Could you check a few things on this model? Use its own coordinates, in mm. A direction names the side the tool comes from. Round coordinates to 2 decimals unless told otherwise and drop trailing zeros. Order: outer loops, then holes, each group sorted by start corner. A loop starts at its lowest first (then second) coordinate and runs counter-clockwise, first axis right, second up. Notation, with made-up numbers: M 80,79.25 L 86,79.25 A17 cw 86,110.25 Z; hole C 69.25,-35.5 d10. An arc over 180 degrees is marked long. Write each question's results on one line, items separated by ' | '. Start each with the question number.
1. We'd pull the mould along Y, two halves only. Please class faces 3 (the flat face through (-7.8, 57.8, -3.9)), 4 (the flat face through (0, 122, -2)), 5 (the flat face through (-71, 240, -2)): released by +Y, released by -Y, zero draft, split by the parting line, or undercut.
2. Suppose I cut it at A-A on z = -1. Give the number of separate pieces and of enclosed holes in the cut face, and give its area (3 significant figures).
3. Please list where these lines run through material, in increasing order: L1, parallel to X at y = 180, z = -2.1; L2, parallel to X at y = 180, z = -4.5; L3, parallel to Y at x = -54.5, z = -1.35.
4. I'm going to push a flat-ended pin straight in: pin 1 (5 mm diameter, centred on x = -69, y = 10, fed in from +Z). Where does the tip first touch, or does it pass through?
5. For faces 1 (the cylindrical face through (-71.5, 225.23, -1.98)), 2 (the cylindrical face through (-71.432, 190.906, -2.465)), which set-ups out of +Z, -Z, +X, -X, +Y, -Y let a thin tool reach every point of the face, with its end or its side?
6. Suppose I cut it at B-B on y = 230. Write out the boundary of the cut face in (x, z), and give its area (3 significant figures).
Autodesk Inventor part; units mm, degrees
ref_plane "Arbeitsebene1" through (-140, 120, 0) normal (0, 1, 0) x (1, 0, 0)
ref_plane "YZ Plane" through (0, 0, 0) normal (1, 0, 0) x (0, 1, 0)
ref_plane "XZ Plane" through (0, 0, 0) normal (0, 1, 0) x (-1, 0, 0)
sketch "Skizze3" plane through (0, 0, 0) normal (0, 0, 1) x (1, 0, 0)
  line L0 (0, 0) -> (-140, 0)
  line L1 (-140, 0) -> (-140, 120)
  line L2 (-140, 240) -> (0, 240)
  line L3 (0, 240) -> (0, 0)
  line L4 (-34.5565, 44.5) -> (-109.2584, 44.5) construction
  line L5 (-42.5521, 75.5) -> (-110.6291, 75.5) construction
  line L6 (-85.5, 104.3529) -> (-85.5, 36.2759) construction
  line L7 (-54.5, 102.2969) -> (-54.5, 32.1639) construction
  line L8 (-70, -15.9958) -> (-70, 12.0858) construction
  circle A0 centre (-70, 60) radius 11
  circle A1 centre (-85.5, 75.5) radius 1.5
  circle A2 centre (-85.5, 44.5) radius 1.5
  circle A3 centre (-54.5, 44.5) radius 1.5
  circle A4 centre (-54.5, 75.5) radius 1.5
  line L9 (-140, 120) -> (0, 120) construction
  line L10 (-140, 120) -> (-140, 240)
  line L11 (-148.6913, 60) -> (9.8942, 60) construction
  line L12 (-160.7703, 180) -> (-4.1331, 180) construction
  point P0 (-70, 0)
  point P1 (-70, 10)
  point P2 (-130, 60)
  point P3 (-140, 180)
  point P4 (-140, 60)
  point P5 (-130, 180)
  point P6 (-10, 180)
  point P7 (-10, 60)
  point P8 (-70, 230)
  dimension "d4" = 240
  dimension "d5" = 140
  dimension "d6" = 31
  dimension "d7" = 31
  dimension "d8" = 15.5
  dimension "d9" = 15.5
  dimension "d10" = 60
  dimension "d11" = 22
  dimension "d12" = 3
  dimension "d13" = 3
  dimension "d14" = 3
  dimension "d15" = 3
  dimension "d22" = 10
  dimension "d23" = 10
  dimension "d24" = 10
  dimension "d25" = 10
  dimension "d26" = 10
  dimension "d34" = 10
extrude "Extrusion3" add sketch "Skizze3" against normal blind 5 contours L0 L1 L10 L2 L3 | A0 | A1 | A2 | A3 | A4
fillet "Rundung1" radius 2 4 edges at (0, 0, -2.5) (0, 240, -2.5) (-140, 240, -2.5) (-140, 0, -2.5)
ref_plane "Arbeitsebene1" through (-140, 120, 0) normal (0, 1, 0) x (1, 0, 0)
extrude "Extrusion4" cut sketch "Skizze3" against normal through all contours A0 | A1 | A2 | A3 | A4
mirror "Spiegeln1" about plane through (-140, 120, 0) normal (0, 1, 0) of "Extrusion4"
hole "Bohrung1" at (-70, 60, 0) at (-70, 10, 0) at (-130, 60, 0) at (-130, 180, 0) at (-10, 180, 0) at (-10, 60, 0) at (-70, 230, 0) direction (0, 0, -1) diameter 5.5 end through all counterbore diameter 10 counterbore depth 3.9
properties part number "BT001_trajan20_21"
Filled sheet:
1) face 3: undercut | face 4: zero draft | face 5: released by +Y
2) separate pieces: 1 | enclosed holes: 16 | area: 32,300 mm^2
3) L1: x = -140 to -135, -125 to -81, -59 to -15, -5 to 0 | L2: x = -140 to -132.75, -127.25 to -81, -59 to -12.75, -7.25 to 0 | L3: y = 0 to 43, 46 to 74, 77 to 163, 166 to 194, 197 to 240
4) pin 1: stops at z = -3.9
5) face 1: +Z | face 2: +Z, -Z
6) outline: M -140,-5 L -72.75,-5 L -72.75,-3.9 L -75,-3.9 L -75,0 L -140,0 Z; M -67.25,-5 L 0,-5 L 0,0 L -65,0 L -65,-3.9 L -67.25,-3.9 Z | area: 655 mm^2
